The figure shows three views and two pictorial views of one solid part (mm, origin at its lowest corner). Answer the questions. Give positions to 0.01 mm unless a question says otherwise; leave off trailing zeros. Order: outer loops, then holes, each group sorted by start corner. A loop starts at its lowest first (then second) coordinate and runs counter-clockwise, first axis right, second up. Notation, with made-up numbers: M -18,51 L 29,51 A26 cw 29,75 Z; hole C -22.5,-14.75 d11. An arc over 180 degrees is marked long. One line per item, written item: value.
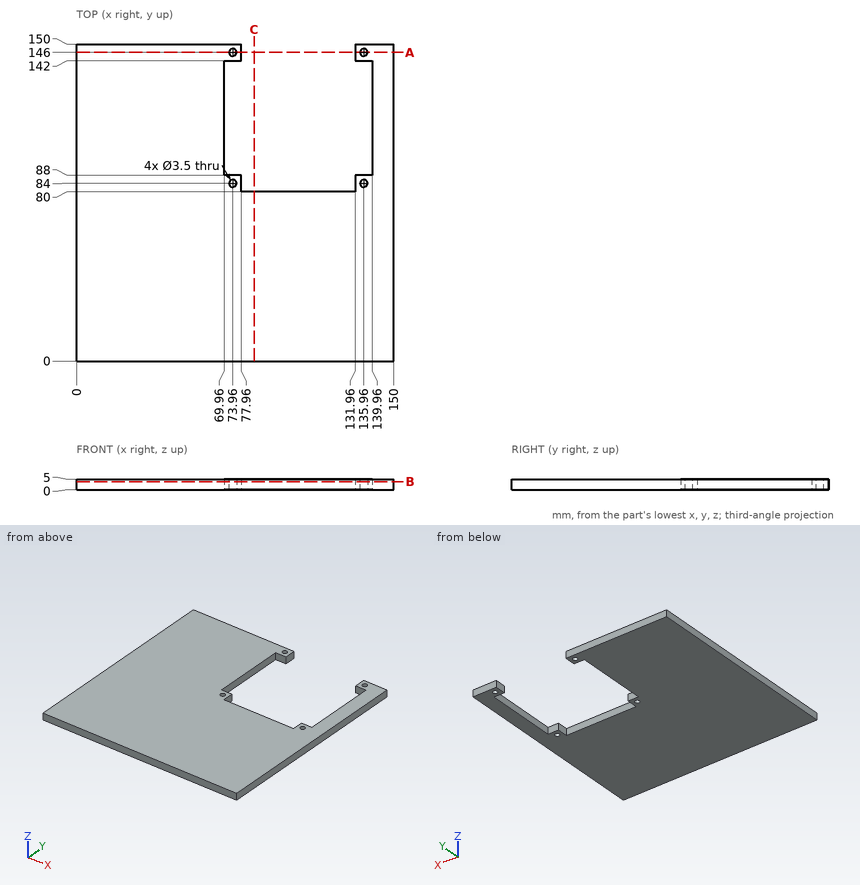
1) Consider probe 1 along X at (y, z) = (84, 3.45); probe 2 along X at (y, z) = (90.5, 0.25); probe 3 along Y at (x, z) = (135, 4.5). Determine where each line is inside the solid, lowest interval first.
Reported:
probe 1: x = 0 to 72.21, 75.71 to 77.96, 131.96 to 134.21, 137.71 to 150
probe 2: x = 0 to 69.96, 139.96 to 150
probe 3: y = 0 to 82.54, 85.46 to 88, 142 to 144.54, 147.46 to 150
2) Find section C-C, the plane x = 84. Write down the section's boundary in (y, z).
Reported:
outline: M 0,0 L 80,0 L 80,5 L 0,5 Z
3) Find section B-B, the plane z = 3.8. Write down the section's boundary in (x, y).
Reported:
outline: M 0,0 L 150,0 L 150,150 L 131.96,150 L 131.96,142 L 139.96,142 L 139.96,88 L 131.96,88 L 131.96,80 L 77.96,80 L 77.96,88 L 69.96,88 L 69.96,142 L 77.96,142 L 77.96,150 L 0,150 Z; hole C 73.96,84 d3.5; hole C 73.96,146 d3.5; hole C 135.96,84 d3.5; hole C 135.96,146 d3.5
4) Find section A-A, the plane y = 146. Write down the section's boundary in (x, z).
Reported:
outline: M 0,0 L 72.21,0 L 72.21,5 L 0,5 Z; M 75.71,0 L 77.96,0 L 77.96,5 L 75.71,5 Z; M 131.96,0 L 134.21,0 L 134.21,5 L 131.96,5 Z; M 137.71,0 L 150,0 L 150,5 L 137.71,5 Z
5) This flat-tipped pin is pushed along its axis until it touches: pin 1 Ø2 at (x, y) = (73.96, 146) entering from +Z. Where does it stop, or does it pass through?
Reported:
pin 1: passes through
